from build123d import *

# Parameters (mm, degrees)
SKETCH1_W           = 40
SKETCH1_H           = 37
BOSS_EXTRUDE1_DEPTH = 20
SKETCH2_W           = 6.5
SKETCH2_H           = 3
BOSS_EXTRUDE2_DEPTH = 20
BOSS_EXTRUDE3_DEPTH = 8.7
BOSS_EXTRUDE4_DEPTH = 3
CUT_EXTRUDE2_REACH  = 67.639
SKETCH5_R           = 2.5


with BuildPart() as part:
    # Sketch1 → Boss-Extrude1 (new body)
    with BuildSketch(Plane.XY):
        with Locations((20, -18.5)):
            Rectangle(SKETCH1_W, SKETCH1_H)
    extrude(amount=BOSS_EXTRUDE1_DEPTH)

    # Sketch2 → Boss-Extrude2 (add)
    with BuildSketch(Plane.XY.offset(20)):
        with Locations((-3.25, -9)):
            Rectangle(SKETCH2_W, SKETCH2_H)
        with Locations((43.25, -9)):
            Rectangle(SKETCH2_W, SKETCH2_H)
    extrude(amount=-BOSS_EXTRUDE2_DEPTH)

    # Sketch3 → Boss-Extrude3 (add)
    with BuildSketch(Plane(origin=(0, 8.7, 0), x_dir=(1, 0, 0), z_dir=(0, 1, 0))):
        with BuildLine():
            ThreePointArc((24.5, -10), (30.5, -16), (36.5, -10))
            Line((36.5, -10), (24.5, -10))
        make_face()
        with BuildLine():
            Line((24.5, -10), (36.5, -10))
            ThreePointArc((36.5, -10), (30.5, -4), (24.5, -10))
        make_face()
    extrude(amount=-BOSS_EXTRUDE3_DEPTH)

    # Sketch4 → Boss-Extrude4 (add)
    with BuildSketch(Plane(origin=(0, 8.7, 0), x_dir=(1, 0, 0), z_dir=(0, 1, 0))):
        with BuildLine():
            Line((33.981730745, -34.857142857), (36.468681277, -10.612244898))
            ThreePointArc((36.468681277, -10.612244898), (30.5, -4), (24.531318723, -10.612244898))
            Line((24.531318723, -10.612244898), (27.018269255, -34.857142857))
            ThreePointArc((27.018269255, -34.857142857), (30.5, -38), (33.981730745, -34.857142857))
        make_face()
    extrude(amount=-BOSS_EXTRUDE4_DEPTH)

    # Sketch5 → Cut-Extrude2 (cut, up to next)
    with BuildSketch(Plane.XZ.offset(10.5), mode=Mode.PRIVATE) as cut_extrude2_sk1:
        with Locations(Location((43.25, 15, 0), (0, 0, 270))):
            Circle(SKETCH5_R)
    cut_extrude2_tool1 = extrude(cut_extrude2_sk1.sketch, amount=-CUT_EXTRUDE2_REACH, mode=Mode.PRIVATE) & part.part
    # Sketch5 → Cut-Extrude2 (cut, up to next)
    with BuildSketch(Plane.XZ.offset(10.5), mode=Mode.PRIVATE) as cut_extrude2_sk2:
        with Locations(Location((43.25, 5, 0), (0, 0, 270))):
            Circle(SKETCH5_R)
    cut_extrude2_tool2 = extrude(cut_extrude2_sk2.sketch, amount=-CUT_EXTRUDE2_REACH, mode=Mode.PRIVATE) & part.part
    # Sketch5 → Cut-Extrude2 (cut, up to next)
    with BuildSketch(Plane.XZ.offset(10.5), mode=Mode.PRIVATE) as cut_extrude2_sk3:
        with Locations(Location((-3.25, 15, 0), (0, 0, 270))):
            Circle(SKETCH5_R)
    cut_extrude2_tool3 = extrude(cut_extrude2_sk3.sketch, amount=-CUT_EXTRUDE2_REACH, mode=Mode.PRIVATE) & part.part
    # Sketch5 → Cut-Extrude2 (cut, up to next)
    with BuildSketch(Plane.XZ.offset(10.5), mode=Mode.PRIVATE) as cut_extrude2_sk4:
        with Locations(Location((-3.25, 5, 0), (0, 0, 270))):
            Circle(SKETCH5_R)
    cut_extrude2_tool4 = extrude(cut_extrude2_sk4.sketch, amount=-CUT_EXTRUDE2_REACH, mode=Mode.PRIVATE) & part.part
    add(cut_extrude2_tool1.solids().sort_by_distance((43.25, -10.5, 15))[0], mode=Mode.SUBTRACT)
    add(cut_extrude2_tool2.solids().sort_by_distance((43.25, -10.5, 5))[0], mode=Mode.SUBTRACT)
    add(cut_extrude2_tool3.solids().sort_by_distance((-3.25, -10.5, 15))[0], mode=Mode.SUBTRACT)
    add(cut_extrude2_tool4.solids().sort_by_distance((-3.25, -10.5, 5))[0], mode=Mode.SUBTRACT)


solid = part.part
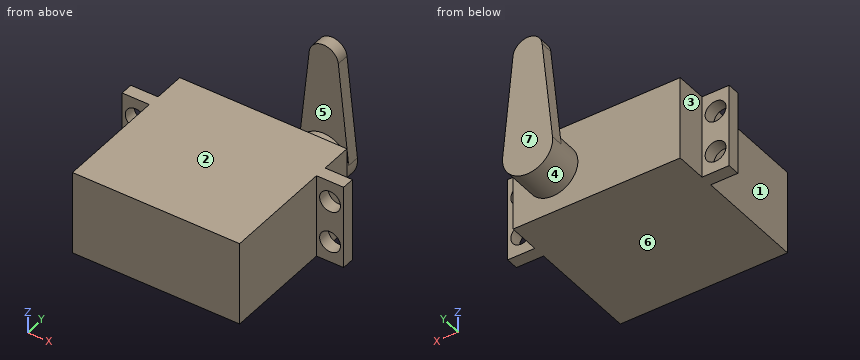
Verification items for the finished model (mm, model axes). Face numbers are marked on the shaded views. A direction names the side the tool comes from. Coordinates: 2 decimals unless noted, no trailing zeros. Loops run counter-clockwise (first coordinate to the right, second up) from the corner with the lowest first, then second, coordinate; pieces in that order, holes last. Notation, with made-up numbers: (84.25, -6) -> (103.25, -6) arc R26 ccw to (103.25, 29) -> close; hole circle Ø6 at (60.5, 75). An arc over 180 degrees is marked (long way). Answer as a JSON object with one key per item and string values. Group by question number.
Item 1: Sectioned sample at C-C on x = 30.5. Record the boundary of the cut face in (y, z).
Item 2: Scan lines: probe 1 along X at (y, z) = (-9.35, 5); probe 2 along Z at (x, y) = (-3, -8); probe 3 along X at (y, z) = (-8, 13). Record each from-to range of solid material in increasing order.
Item 3: Sectioned sample at D-D on y = -5.5. Record the boundary of the cut face in (x, z), plus the area to 3 significant figures.
Item 4: Tool access check on the marked faces 1, 2 and 3. Record the directions out of +Z, -Z, +X, -X, +Y, -Y that give a thin tool (end or side, any length) a straight path to the whole face; none if there is none.
Item 5: Mould release check, pull along Y, two halves, no side actions. Record for the marked faces 4, 5, 6 and 7: +Y half, -Y half, draft (parallel to the pull), parting line (faces both ways), or undercut.
Item 6: Sectioned sample at B-B on z = 5. Record the boundary of the cut face in (x, y).
Item 7: Sectioned sample at A-A on x = 43.25. Record the boundary of the cut face in (y, z), plus the area to 3 significant figures.
Item 8: Depth check by flat-ended pin: pin 1 (11 mm diameter, centred on x = 19, y = -13, fed in from +Z); pin 2 (10 mm diameter, centred on x = 12.5, z = 8, fed in from +Y); pin 3 (16 mm diameter, centred on y = -21.5, z = 13, fed in from -X); pin 4 (2 mm diameter, centred on x = 42.5, z = 14, fed in from +Y). Enter the tip coordinate at first touch or a pass-through.
Evaluation:
{
 "1": {"outline": "(-37, 0) -> (0, 0) -> (0, 4) -> (8.7, 4) -> (8.7, 38) -> (5.7, 38) -> (5.7, 16) -> (0, 16) -> (0, 20) -> (-37, 20) -> close"},
 "2": {"probe 1": "x = -6.5 to -5.75, -0.75 to 40.75, 45.75 to 46.5", "probe 2": "z = 0 to 2.51, 7.49 to 12.51, 17.49 to 20", "probe 3": "x = -6.5 to -4.75, -1.75 to 41.75, 44.75 to 46.5"},
 "3": {"outline": "(0, 0) -> (40, 0) -> (40, 20) -> (0, 20) -> close", "area": "800 mm²"},
 "4": {"face 1": "+Z, -Z, -X, -Y", "face 2": "+Z, +X, -X, -Y", "face 3": "+Z, -Z, -X, +Y"},
 "5": {"face 4": "undercut", "face 5": "undercut", "face 6": "draft", "face 7": "+Y half"},
 "6": {"outline": "(-6.5, -10.5) -> (-5.75, -10.5) -> (-5.75, -7.5) -> (-6.5, -7.5) -> close; (-0.75, -10.5) -> (0, -10.5) -> (0, -37) -> (40, -37) -> (40, -10.5) -> (40.75, -10.5) -> (40.75, -7.5) -> (40, -7.5) -> (40, 0) -> (33.82, 0) -> (33.82, 8.7) -> (27.18, 8.7) -> (27.18, 0) -> (0, 0) -> (0, -7.5) -> (-0.75, -7.5) -> close; (45.75, -10.5) -> (46.5, -10.5) -> (46.5, -7.5) -> (45.75, -7.5) -> close"},
 "7": {"outline": "(-10.5, 0) -> (-7.5, 0) -> (-7.5, 2.5) -> (-10.5, 2.5) -> close; (-10.5, 7.5) -> (-7.5, 7.5) -> (-7.5, 12.5) -> (-10.5, 12.5) -> close; (-10.5, 17.5) -> (-7.5, 17.5) -> (-7.5, 20) -> (-10.5, 20) -> close", "area": "30.0 mm²"},
 "8": {"pin 1": "stops at z = 20", "pin 2": "stops at y = 0", "pin 3": "stops at x = 0", "pin 4": "passes through"}
}
